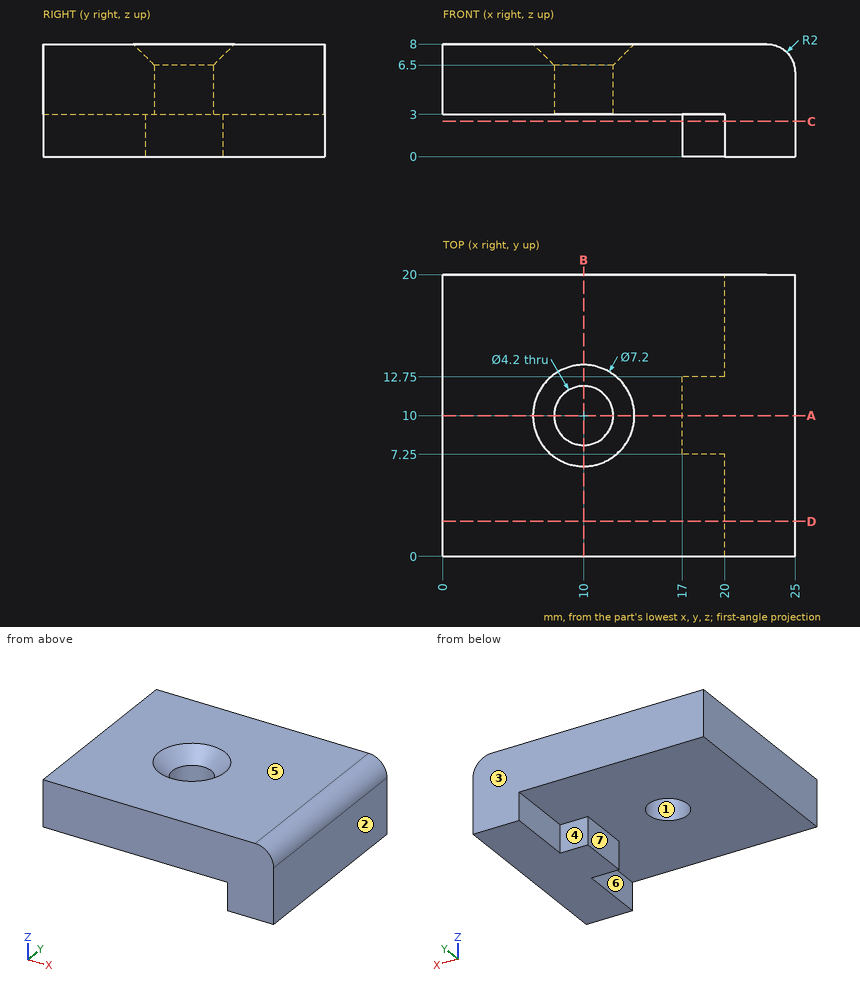
Job drawing, mm, ordinate dimensions from the low corner. One solid piece. A direction names the side the tool comes from. Coordinates: 2 decimals unless noted, no trailing zeros. Order: outer loops, then holes, each group sorted by start corner. A loop starts at its lowest first (then second) coordinate and runs counter-clockwise, first axis right, second up. Notation, with made-up numbers: (25.5, 83.5) - (33.5, 83.5) arc R15 cw to (33.5, 102.5) - close; hole circle Ø1 at (4.5, -4). An arc over 180 degrees is marked (long way). Use CSV: the item, a comma, the result in double quotes.
Item 1: Probe probe 1 along Y at (x, z) = (10, 5.5); probe 2 along X at (y, z) = (1, 1); probe 3 along Z at (x, y) = (17, 5.75). List the from-to ranges inside material, lowest first.
Solved:
probe 1,"y = 0 to 7.9, 12.1 to 20"
probe 2,"x = 20 to 25"
probe 3,"z = 3 to 8"
Item 2: Saw through at C-C on z = 2.5. Give the cut face in (x, y), and give its area (4 significant figures).
Solved:
outline,"(17, 7.25) - (20, 7.25) - (20, 0) - (25, 0) - (25, 20) - (20, 20) - (20, 12.75) - (17, 12.75) - close"
area,"116.5 mm²"
Item 3: Drop flat-ended pins along their axis: P1, Ø1, axis at x = 13, z = 6.5, coming from the -Y side; P2, Ø1.5, axis at x = 19, z = 1.5, coming from the -Y side; P3, Ø3.5, axis at y = 4, z = 1, coming from the -X side; P4, Ø1.5, axis at x = 19, z = 1, coming from the +Y side. Give the stop position or say it passes through.
Solved:
P1,"stops at y = 0"
P2,"stops at y = 7.25"
P3,"stops at x = 20"
P4,"stops at y = 12.75"
Item 4: Mould opens along X. For the marked faces 1, 2 and 3 say: +X half, -X half, draft (parallel to the pull), parting line (faces both ways), or undercut.
Solved:
face 1,"undercut"
face 2,"+X half"
face 3,"draft"
Item 5: Saw through at B-B on x = 10. Give the cut face in (y, z), and give its area (4 significant figures).
Solved:
outline,"(0, 3) - (7.9, 3) - (7.9, 6.5) - (6.4, 8) - (0, 8) - close; (12.1, 3) - (20, 3) - (20, 8) - (13.6, 8) - (12.1, 6.5) - close"
area,"76.75 mm²"
Item 6: Saw through at D-D on y = 2.5. Give the cut face in (x, z), and give its area (3 significant figures).
Solved:
outline,"(0, 3) - (20, 3) - (20, 0) - (25, 0) - (25, 6) arc R2 ccw to (23, 8) - (0, 8) - close"
area,"139 mm²"
Item 7: 3-axis set-ups, long thin cutter, end or side, ignore diameter. For the marked faces 4, 5, 6 and 7: which of +Z, -Z, +X, -X, +Y, -Y reach the whole face in a straight line?
Solved:
face 4,"-Z, -X, +Y"
face 5,"+Z, +X, -X, +Y, -Y"
face 6,"-Z, -X, -Y"
face 7,"-Z, -X, +Y, -Y"
Item 8: Saw through at A-A on y = 10. Give the cut face in (x, z), and give its area (3 significant figures).
Solved:
outline,"(0, 3) - (7.9, 3) - (7.9, 6.5) - (6.4, 8) - (0, 8) - close; (12.1, 3) - (17, 3) - (17, 0) - (25, 0) - (25, 6) arc R2 ccw to (23, 8) - (13.6, 8) - (12.1, 6.5) - close"
area,"125 mm²"
